CAD build for the part. Positions are in the model's coordinates, mm. Face numbers are marked on the shaded views. A direction names the side the tool comes from. Coordinates: 2 decimals unless noted, no trailing zeros. Loops run counter-clockwise (first coordinate to the right, second up) from the corner with the lowest first, then second, coordinate; pieces in that order, holes last. Notation, with made-up numbers: (64.5, 6) - (77.5, 6) arc R25 ccw to (77.5, 22) - close; hole circle Ø4 at (12.5, -9.75). An arc over 180 degrees is marked (long way). Put each result on its own line as item: value.
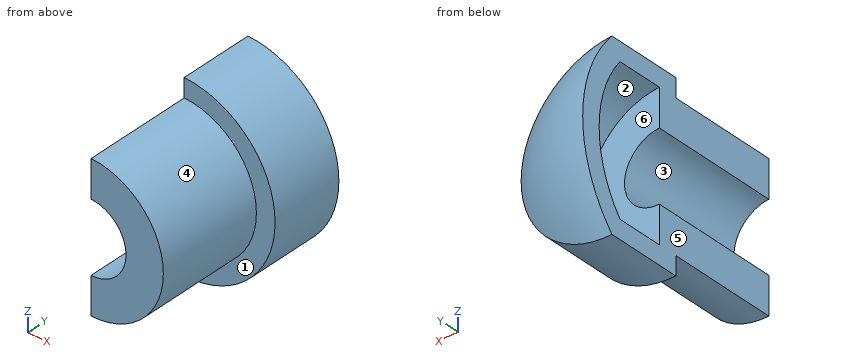
```python
from build123d import *

# Parameters (mm, degrees)
SKETCH1_R           = 2.9
BOSS_EXTRUDE1_DEPTH = 5
CUT_EXTRUDE1_REACH  = 8.467
SKETCH2_R           = 1.4
CUT_EXTRUDE2_REACH  = 11.945
SKETCH8_W           = 3.65
SKETCH8_H           = 7.3


with BuildPart() as part:
    # Sketch1 → Boss-Extrude1 (new body)
    with BuildSketch(Plane(origin=(0, 0, 0), x_dir=(1, 0, 0), z_dir=(0, 1, 0))):
        with Locations(Location((0, 0, 0), (0, 0, 270))):
            Circle(SKETCH1_R)
    extrude(amount=BOSS_EXTRUDE1_DEPTH)

    # Sketch2 → Cut-Extrude1 (cut, up to next)
    with BuildSketch(Plane(origin=(0, 5, 0), x_dir=(1, 0, 0), z_dir=(0, 1, 0)), mode=Mode.PRIVATE) as cut_extrude1_sk1:
        with Locations(Location((0, 0, 0), (0, 0, 270))):
            Circle(SKETCH2_R)
    cut_extrude1_tool1 = extrude(cut_extrude1_sk1.sketch, amount=-CUT_EXTRUDE1_REACH, mode=Mode.PRIVATE) & part.part
    add(cut_extrude1_tool1.solids().sort_by_distance((0, 5, 0))[0], mode=Mode.SUBTRACT)

    # Sketch6 → Revolve2 (revolve)
    with BuildSketch(Plane.XY):
        with BuildLine():
            Line((2.9, 6.8), (2.9, 5))
            Line((2.9, 5), (2.9, 4.25))
            Line((2.9, 4.25), (3.65, 4.25))
            Line((3.65, 4.25), (3.65, 5))
            Line((3.65, 5), (3.65, 7.163179564))
            ThreePointArc((3.65, 7.163179564), (1.943552731, 8.155281325), (0, 8.5))
            Line((0, 8.5), (0, 7.75))
            ThreePointArc((0, 7.75), (1.525819452, 7.506448853), (2.9, 6.8))
        make_face()
    revolve(axis=Axis((0, 5, 0), (0, 1, 0)))

    # Sketch8 → Cut-Extrude2 (cut, up to next)
    with BuildSketch(Plane(origin=(0, 0, 0), x_dir=(1, 0, 0), z_dir=(0, 1, 0)), mode=Mode.PRIVATE) as cut_extrude2_sk1:
        with Locations((-1.825, 0)):
            Rectangle(SKETCH8_W, SKETCH8_H)
    cut_extrude2_tool1 = extrude(cut_extrude2_sk1.sketch, amount=CUT_EXTRUDE2_REACH, mode=Mode.PRIVATE) & part.part
    add(cut_extrude2_tool1.solids().sort_by_distance((-1.825, 0, 0))[0], mode=Mode.SUBTRACT)


solid = part.part
```
Q1. Pin check, flat tips, straight feed: pin 1 Ø2 at (x, y) = (2.5, 2.5) entering from -Z; pin 2 Ø1 at (y, z) = (6, -2.5) entering from +X; pin 3 Ø2 at (y, z) = (2, 2) entering from +X. Stop position of each tip, or through.
Determined:
pin 1: z = -2.48
pin 2: x = 3.05
pin 3: x = 2.72
Q2. Mould opens along Z. For the marked faces 4, 5 and 6 say: +Z half, -Z half, draft (parallel to the pull), parting line (faces both ways), or undercut.
Determined:
face 4: parting line
face 5: draft
face 6: undercut
Q3. Wall check: L1, parallel to Y at x = 1.6, z = 1.25; L2, parallel to X at y = 6.25, z = 0; L3, parallel to Y at x = 0.8, z = 2.5. Give the ranges that are in metal, low to high. Write a range as from..to.
Determined:
L1: 0..5, 7.31..8.12
L2: 2.9..3.65
L3: 0..5, 6.99..7.85
Q4. Slice it at A-A, the plane z = 0. Give the cut face in (x, y), then the cut area to 3 significant figures.
Determined:
outline: (0, 7.75) arc R4.9 cw to (2.9, 6.8) - (2.9, 5) - (1.4, 5) - (1.4, 0) - (2.9, 0) - (2.9, 4.25) - (3.65, 4.25) - (3.65, 7.16) arc R5.65 ccw to (0, 8.5) - close
area: 12.2 mm2
Q5. Tool access for the marked faces 1, 2 and 3: list every direction of +Z, -Z, +X, -X, +Y, -Y with a clear straight run to the whole face (end or side of a thin tool).
Determined:
face 1: +X, -Y
face 2: -X
face 3: -X, -Y
Q6. Slice it at C-C, the plane y = 5.25. Give the cut face in (x, z), then the cut area to 3 significant figures.
Determined:
outline: (0, -3.65) arc R3.65 ccw to (0, 3.65) - (0, 2.9) arc R2.9 cw to (0, -2.9) - close
area: 7.72 mm2
Q7. Slice it at D-D, the plane z = 2.5. Give the cut face in (x, y), then the cut area to 3 significant figures.
Determined:
outline: (0, 0) - (1.47, 0) - (1.47, 4.25) - (2.66, 4.25) - (2.66, 7.16) arc R5.07 ccw to (0, 7.92) - (0, 7.06) arc R4.22 cw to (1.47, 6.8) - (1.47, 5) - (0, 5) - close
area: 12.4 mm2
Q8. Slice it at B-B, the plane x = 0.55. Give the cut face in (y, z), then the cut area to 3 significant figures.
Determined:
outline: (0, -2.85) - (4.25, -2.85) - (4.25, -3.61) - (7.16, -3.61) arc R5.62 ccw to (7.16, 3.61) - (4.25, 3.61) - (4.25, 2.85) - (0, 2.85) - (0, 1.29) - (5, 1.29) - (5, 2.85) - (6.8, 2.85) arc R4.87 cw to (6.8, -2.85) - (5, -2.85) - (5, -1.29) - (0, -1.29) - close
area: 25.0 mm2
